from build123d import *

# Parameters (mm, degrees)
F1_DEPTH      = 12.5
F4_DEPTH      = 12.5
F4_DEPTH_BACK = 12.5
F6_DEPTH      = 78.7353324739
F7_W          = 25
F7_H          = 22.2357761898
F8_DEPTH      = 5


with BuildPart() as f1:
    # F0 (on Right) → F1 (new body, symmetric)
    with BuildSketch(Plane.YZ):
        Polygon((-34, 0), (0, 0), (0, 72.9132352973), align=None)
    extrude(amount=F1_DEPTH, both=True)

    # F3 (on Right) → F4 (cut, two sides)
    with BuildSketch(Plane.YZ) as f4_sk:
        with BuildLine():
            ThreePointArc((0, 16.5421399337), (-7.9228514216, 9.7223765395), (-11.7642238102, 0))
            Line((-11.7642238102, 0), (0, 0))
            Line((0, 0), (0, 16.5421399337))
        make_face()
    extrude(amount=-F4_DEPTH, mode=Mode.SUBTRACT)
    extrude(f4_sk.sketch, amount=F4_DEPTH_BACK, mode=Mode.SUBTRACT)

    # F5 (on face) → F6 (cut, up to face)
    with BuildSketch(Plane(origin=(0, 27.9273893647, 59.8904797643), x_dir=(1, 0, 0), z_dir=(0, 0.4226182617, 0.906307787))):
        with BuildLine():
            Line((-8, 3.5331053375), (-8, -16.9910104243))
            ThreePointArc((-8, -16.9910104243), (0, -24.9910104243), (8, -16.9910104243))
            Line((8, -16.9910104243), (8, 3.5331053375))
            Line((8, 3.5331053375), (-8, 3.5331053375))
        make_face()
    extrude(amount=-F6_DEPTH, mode=Mode.SUBTRACT)

    # F7 (on face) → F8 (join)
    with BuildSketch(Plane(origin=(0, 0, 0), x_dir=(1, 0, 0), z_dir=(0, 0, -1))):
        with Locations((0, 22.8821119051)):
            Rectangle(F7_W, F7_H)
    extrude(amount=F8_DEPTH)


solid = f1.part
Geometry: final body of the model. Coordinates: model frame, mm. A direction names the side the tool comes from. Round coordinates to 2 decimals unless told otherwise and drop trailing zeros. Loops run counter-clockwise (first coordinate to the right, second up) from the corner with the lowest first, then second, coordinate; pieces in that order, holes last. Notation, with made-up numbers: M 80,81.5 L 86,81.5 A28 cw 86,103.5 Z; hole C 84.5,-2.75 d5. An arc over 180 degrees is marked long. One line per question, with ' | ' between items.
(1) Contact query for flat-ended pins moving along their axis: P1, Ø2, axis at x = 7, y = -9.5, coming from the +Z side; P2, Ø1.5, axis at x = 4, z = 60.5, coming from the -Y side; P3, Ø5.5, axis at x = -4, z = -3.5, coming from the +Y side. Output: stop coordinate, or through.
Check result:
P1: stops at z = 54.68 | P2: stops at y = -6.14 | P3: stops at y = -11.76
(2) Cut plane C-C on x = -1.5. Return the cut outline in (y, z).
Check result:
outline: M -34,-5 L -11.76,-5 L -11.76,0 L -27.42,0 L 0,58.8 L 0,72.91 L -34,0 Z
(3) Cut plane A-A on x = -8.75. Return the cut outline in (y, z).
Check result:
outline: M -34,-5 L -11.76,-5 L -11.76,0 A21.82 cw 0,16.54 L 0,72.91 L -34,0 Z
(4) Cut plane B-B on z = 62. Return the cut outline in (x, y), plus the area to 3 significant figures.
Check result:
outline: M -12.5,-5.09 L 12.5,-5.09 L 12.5,0 L -12.5,0 Z | area: 127 mm2
(5) Pull-direction query (X, two-part tool) for faces 1 (the cylindrical face through (-10.28, -7.84, 9.84)), 2 (the flat face through (12.5, -13, 26)), 3 (the cylindrical face through (-0.176, -13.592, 29.98)); classes: +X half, -X half, draft (parallel to the pull), parting line (faces both ways), or undercut.
Check result:
face 1: draft | face 2: +X half | face 3: undercut
(6) Material intervals for line 1 along X through (y, z) = (-16.5, 4); line 2 along Z through (x, y) = (4.75, -16); line 3 along Z through (x, y) = (0, -16.5), sorted ascending. Write a range as from..to.
Check result:
line 1: x = -12.5..-8, 8..12.5 | line 2: z = -5..0, 21.12..38.6 | line 3: z = -5..0, 23.75..37.53
(7) Cut plane D-D on x = 6.5. Return the cut outline in (y, z).
Check result:
outline: M -34,-5 L -11.76,-5 L -11.76,0 L -23.89,0 L 0,51.24 L 0,72.91 L -34,0 Z
(8) Access query for faces 4 (the flat face through (0, -34, -2)), 5 (the flat face through (0, -11.764, -2)), 6 (the flat face through (-8, -6, 19)). Directions: +Z, -Z, +X, -X, +Y, -Y. A direction counts if a zero-diameter tool reaches every point of the face in a straight line with its end or side. Return the directions, or none.
Check result:
face 4: +Z, -Z, +X, -X, -Y | face 5: -Z, +X, -X, +Y | face 6: +Y
